The listing builds one solid part. Answer for the finished solid, in the listing's coordinates (mm). A direction names the side the tool comes from. Coordinates: 2 decimals unless noted, no trailing zeros. Write each loop counter-clockwise with the first axis right and the second up, starting at its lowest first coordinate (ties: lowest second). Pieces come first, ordered by that corner, then holes.
```python
from build123d import *

# Parameters (mm, degrees)
F0_W      = 40
F0_H      = 28
F1_DEPTH  = 6
F2_W      = 20
F2_H      = 28
F3_DEPTH  = 25
F5_DEPTH  = 30.001
F7_D      = 4.1
F7_DEPTH  = 12
F7_TIP    = 1.231764269
F9_D      = 5.5
F9_DEPTH  = 12
F9_TIP    = 1.6523667023
F11_D     = 5.5
F11_DEPTH = 12
F11_TIP   = 1.6523667023


with BuildPart() as f1:
    # F0 (on Top) → F1 (new body)
    with BuildSketch(Plane.XY):
        with Locations((20, 14)):
            Rectangle(F0_W, F0_H)
    extrude(amount=F1_DEPTH)

    # F2 (on face) → F3 (join)
    with BuildSketch(Plane.XY.offset(6)):
        with Locations((20, 14)):
            Rectangle(F2_W, F2_H)
    extrude(amount=F3_DEPTH)

    # F4 (on face) → F5 (cut, through all)
    with BuildSketch(Plane(origin=(10, 0, 0), x_dir=(0, -1, 0), z_dir=(-1, 0, 0))):
        with BuildLine():
            Line((-28, 17.5), (-21.9372539332, 17.5))
            ThreePointArc((-21.9372539332, 17.5), (-6, 18.5), (-21.9372539332, 19.5))
            Line((-21.9372539332, 19.5), (-28, 19.5))
            Line((-28, 19.5), (-28, 17.5))
        make_face()
    extrude(amount=-F5_DEPTH, mode=Mode.SUBTRACT)

    # F7 (one way)
    with BuildSketch(Plane.XY.offset(17.5)):
        with Locations((20, 25)):
            Circle(F7_D / 2)
    extrude(amount=-F7_DEPTH, mode=Mode.SUBTRACT)
    with Locations(Plane.XY.offset(17.5)):
        with Locations((20, 25)):
            with Locations((0, 0, -(F7_DEPTH + F7_TIP / 2))):  # 118° drill point
                Cone(0, F7_D / 2, F7_TIP, mode=Mode.SUBTRACT)

    # F9
    with Locations(Plane.XY.offset(31)):
        with Locations((20, 25)):
            Hole(F9_D / 2, depth=F9_DEPTH)
            with Locations((0, 0, -(F9_DEPTH + F9_TIP / 2))):  # 118° drill point
                Cone(0, F9_D / 2, F9_TIP, mode=Mode.SUBTRACT)

    # F11
    with Locations(Plane.XY.offset(6)):
        with Locations((5, 5), (5, 23), (35, 23), (35, 5)):
            Hole(F11_D / 2, depth=F11_DEPTH)
            with Locations((0, 0, -(F11_DEPTH + F11_TIP / 2))):  # 118° drill point
                Cone(0, F11_D / 2, F11_TIP, mode=Mode.SUBTRACT)


solid = f1.part
```
(1) Section A-A, the plane x = 5 is taken. Write down the section's boundary in (y, z).
(2) Section D-D, the plane z = 20.5 is taken. Write down the section's boundary in (x, y).
(3) Each of these flat-tipped pins is pushed along its axis until it touches: pin 1 (3.5 mm diameter, centred on x = 35, y = 23, fed in from -Z); pin 2 (8 mm diameter, centred on x = 2.5, y = 10, fed in from +Z); pin 3 (1.5 mm diameter, centred on y = 23, z = 26, fed in from +X); pin 4 (12.5 mm diameter, centred on y = 12, z = 19, fed in from -X). Where does it stop, or does it pass through?
(4) Which of the six approach directions +Z, -Z, +X, -X, +Y, -Y give full straight-line access (tool end or side, diameter ignored) to faces 1 (the flat face through (5, 14, 6)), 2 (the flat face through (17.6, 22.9, 19.5)), 3 (the cylindrical face through (18.5, 26.4, 11.6))?
(5) Section C-C, the plane x = 28 is taken. Write down the section's boundary in (y, z).
(6) For a pull along X with two mould halves and no side action, classify faces 4 (the flat face through (30, 7.6, 12.8)), 5 (the conical face through (19.644, 25.016, 4.482)), 6 (the flat face through (0, 14, 3)), 7 (the flat face through (20, 14, 31)) as pulls with the +X half, pulls with the -X half, needs draft (parallel to the pull), parting line crosses it, or undercut.
(7) Find the intervals of material crossed by probe 1 along Y at (x, z) = (5, 1.7); probe 2 along Z at (x, y) = (26, 13.75); probe 3 along Y at (x, z) = (20, 20), in increasing order.
(8) Section B-B, the plane y = 9.75 is taken. Write down the section's boundary in (x, z).
Solution:
1. outline: (0, 0) - (2.25, 0) - (2.25, 6) - (0, 6) - close; (7.75, 0) - (20.25, 0) - (20.25, 6) - (7.75, 6) - close; (25.75, 0) - (28, 0) - (28, 6) - (25.75, 6) - close
2. outline: (10, 0) - (30, 0) - (30, 6.25) - (10, 6.25) - close; (10, 21.75) - (30, 21.75) - (30, 28) - (10, 28) - close; hole circle Ø5.5 at (20, 25)
3. pin 1: passes through
3. pin 2: stops at z = 6
3. pin 3: stops at x = 30
3. pin 4: stops at x = 10
4. face 1: +Z, -X, +Y, -Y
4. face 2: +X, -X, +Y
4. face 3: +Z
5. outline: (0, 0) - (28, 0) - (28, 17.5) - (21.94, 17.5) arc R8 cw (long way) to (21.94, 19.5) - (28, 19.5) - (28, 31) - (0, 31) - close
6. face 4: pulls with the +X half
6. face 5: undercut
6. face 6: pulls with the -X half
6. face 7: needs draft
7. probe 1: y = 0 to 2.25, 7.75 to 20.25, 25.75 to 28
7. probe 2: z = 0 to 10.5, 26.5 to 31
7. probe 3: y = 0 to 6.14, 21.86 to 22.25, 27.75 to 28
8. outline: (0, 0) - (40, 0) - (40, 6) - (30, 6) - (30, 11.72) - (10, 11.72) - (10, 6) - (0, 6) - close; (10, 25.28) - (30, 25.28) - (30, 31) - (10, 31) - close
